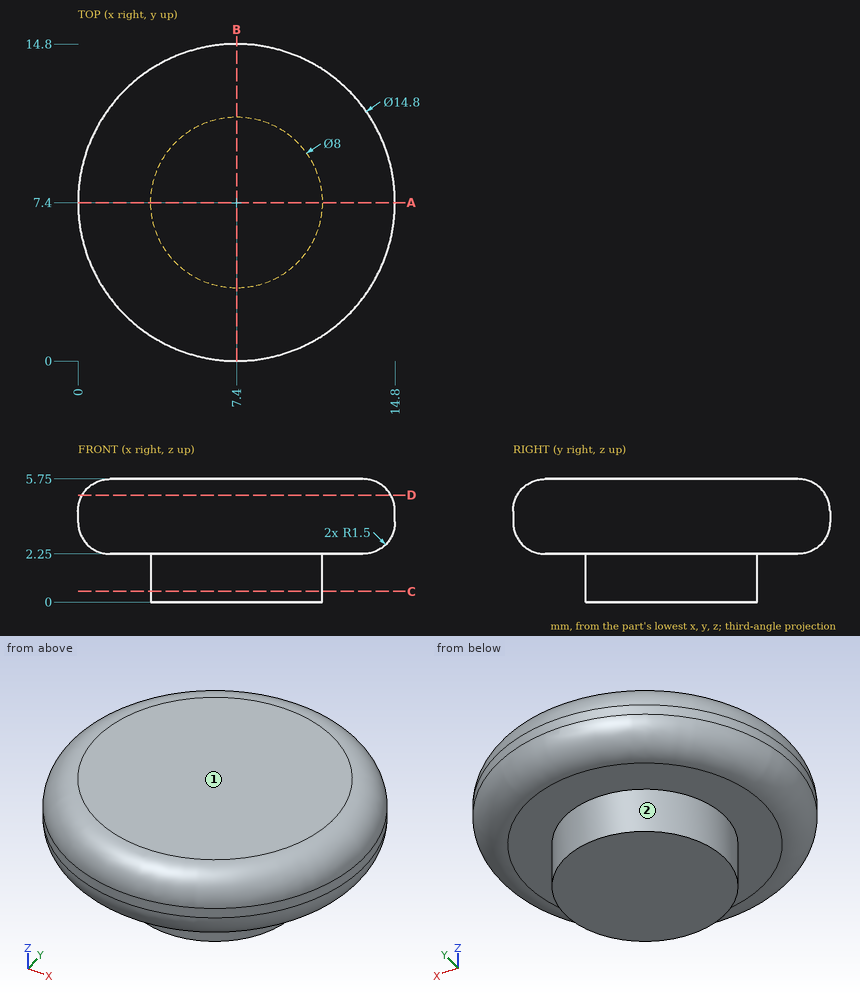
Source: three-view drawing plus pictorial views. Frame: mm from the lowest corner of the part. A direction names the side the tool comes from. Coordinates: 2 decimals unless noted, no trailing zeros. Order: outer loops, then holes, each group sorted by start corner. A loop starts at its lowest first (then second) coordinate and runs counter-clockwise, first axis right, second up.
1) Section D-D (z = 5). Return loops of the section in (x, y), then the cut area to 3 significant figures.
Result sheet:
outline: circle Ø14.4 at (7.4, 7.4)
area: 163 mm2
2) Set-up query: the marked faces 1 and 2. Return all of +Z, -Z, +X, -X, +Y, -Y with unobstructed straight access to the full face (end or side cutting, diameter ignored); none if empty.
Result sheet:
face 1: +Z, +X, -X, +Y, -Y
face 2: -Z
3) Section A-A (y = 7.4). Return loops of the section in (x, z).
Result sheet:
outline: (0, 3.75) arc R1.5 ccw to (1.5, 2.25) - (3.4, 2.25) - (3.4, 0) - (11.4, 0) - (11.4, 2.25) - (13.3, 2.25) arc R1.5 ccw to (14.8, 3.75) - (14.8, 4.25) arc R1.5 ccw to (13.3, 5.75) - (1.5, 5.75) arc R1.5 ccw to (0, 4.25) - close
4) Ray query, probe 1 along Z at (x, y) = (5.5, 12.5); probe 2 along X at (y, z) = (6, 0.35); probe 3 along X at (y, z) = (8.5, 4.7). Return the intervals inside material, ascending.
Result sheet:
probe 1: z = 2.25 to 5.75
probe 2: x = 3.65 to 11.15
probe 3: x = 0.15 to 14.65
5) Section C-C (z = 0.5). Return loops of the section in (x, y).
Result sheet:
outline: circle Ø8 at (7.4, 7.4)
6) First-contact query: P1, Ø2, axis at y = 9, z = 3, coming from the +X side; P2, Ø2, axis at y = 8.5, z = 3.5, coming from the -X side; P3, Ø5, axis at x = 12.5, y = 2.5, coming from the -Z side. Flat tips, straight axial feed; report the tip coordinate or a pass-through.
Result sheet:
P1: stops at x = 14.75
P2: stops at x = 0
P3: stops at z = 2.25
